The model under review builds one solid part; all positions refer to its coordinate system, in mm. A direction names the side the tool comes from. Round coordinates to 2 decimals unless told otherwise and drop trailing zeros. Write each loop counter-clockwise with the first axis right and the second up, starting at its lowest first coordinate (ties: lowest second). Pieces come first, ordered by that corner, then holes. Notation, with made-up numbers: (58.5, 36) - (92.5, 36) arc R30 cw to (92.5, 60) - close; hole circle Ø11 at (35, 46). An arc over 180 degrees is marked (long way). Return JSON: item names as keys, results as strings.
Autodesk Inventor part; units mm, degrees
ref_plane "YZ Plane" through (0, 0, 0) normal (1, 0, 0) x (0, 1, 0)
ref_plane "XZ Plane" through (0, 0, 0) normal (0, 1, 0) x (-1, 0, 0)
ref_plane "XY Plane" through (0, 0, 0) normal (0, 0, 1) x (1, 0, 0)
sketch "Sketch1" plane through (0, 0, 0) normal (0, 0, 1) x (1, 0, 0)
  line L0 (17.5514, 0) -> (46.0756, 0)
  line L1 (46.0756, 0) -> (46.0756, 12.7)
  line L2 (46.0756, 12.7) -> (0, 12.7)
  line L3 (0, 12.7) -> (0, 0)
  line L4 (17.5514, 12.7) -> (17.5514, 0)
  line L5 (46.0756, 8.9662) -> (42.3672, 8.9662)
  line L6 (42.3672, 7.747) -> (42.3672, 0)
  line L7 (46.0756, 7.747) -> (42.3672, 7.747)
  line L8 (46.0756, 8.9662) -> (42.3672, 7.747)
  line L9 (0, 11.1252) -> (0, 12.7)
  line L10 (17.5514, 0) -> (23.85, 0)
  line L11 (0, -2.5) -> (0, 0)
  line L12 (0, 12.7) -> (38.0365, 12.7)
  line L13 (38.0365, 12.7) -> (38.0365, 14.2748)
  line L14 (38.0365, 14.2748) -> (0, 14.2748)
  line L15 (0, 14.2748) -> (0, 12.7)
  line L16 (17.5514, 12.7) -> (17.5514, 14.2748)
  line L17 (0, 0) -> (17.5514, 0)
  dimension "d1" = 12.7
  dimension "d3" = 3.7338
  dimension "d5" = 4.953
  dimension "d8" = 17.5514
  dimension "d9" = 42.3672
  dimension "d10" = 46.0756
  dimension "d11" = 1.5748
  dimension "d12" = 38.0365
revolve "Revolution1" add sketch "Sketch1" angle 360 about axis through (0, 12.7, 0) along (0, -1, 0) contours L4 L2 L1 L8 L6 L0 | L17 L3 L2 L4 | L16 L14 L13 L2 | L2 L15 L14 L16
sketch "Sketch2" plane through (0, 14.2748, 0) normal (0, 1, 0) x (1, 0, 0)
  circle A0 centre (0, 0) radius 30.1752
  point P0 (0, 30.1752)
  point P1 (0, -30.1752)
  dimension "d14" = 60.3504
hole "Hole1" at (0, 14.2748, -30.1752) at (0, 14.2748, 30.1752) direction (0, -1, 0) diameter 6.35 depth 10.16
properties part number "2016.06.09 Blank Adapter"
(1) Add section A-A (x = 0). Write out the cut boundary in (y, z), plus the area to 3 significant figures.
Filled in:
{"outline": "(0, -42.37) - (7.75, -42.37) - (8.97, -46.08) - (12.7, -46.08) - (12.7, -38.04) - (14.27, -38.04) - (14.27, -33.35) - (4.11, -33.35) - (4.11, -27) - (14.27, -27) - (14.27, 27) - (4.11, 27) - (4.11, 33.35) - (14.27, 33.35) - (14.27, 38.04) - (12.7, 38.04) - (12.7, 46.08) - (8.97, 46.08) - (7.75, 42.37) - (0, 42.37) - close", "area": "1,100 mm2"}
(2) For faces 4 (the cylindrical face through (-9.18, 3.82, -41.36)), 5 (the cylindrical face through (-0.954, 9.124, 33.204)), 6 (the flat face through (-1, 14.275, 1)), list the 3-axis set-ups (+Z, -Z, +X, -X, +Y, -Y) from which the entire face can be reached by the end or side of a thin tool; tool diameter is ignored.
Filled in:
{"face 4": "-Y", "face 5": "+Y", "face 6": "+Z, -Z, +X, -X, +Y"}
(3) Wall thickness on line 1 (Z direction, x = 0, y = 9.25); line 2 (Z direction, x = 0, y = 6.75); line 3 (Y direction, x = 13, z = 39): over which ranges is each line inside the solid? List them lowest first.
Filled in:
{"line 1": "z = -46.08 to -33.35, -27 to 27, 33.35 to 46.08", "line 2": "z = -42.37 to -33.35, -27 to 27, 33.35 to 42.37", "line 3": "y = 0 to 12.7"}
(4) Mouldability with a two-part tool opening along Z and no side actions: class faces 1 (the flat face through (-1, 0, 1)), 2 (the flat face through (0, 4.115, 30)), 3 (the cylindrical face through (-9.99, 10.86, 44.98)) as released by +Z, released by -Z, zero draft, split by the parting line, or undercut.
Filled in:
{"face 1": "zero draft", "face 2": "undercut", "face 3": "split by the parting line"}
(5) Add section B-B (y = 5.5). Write out the cut boundary in (x, z) (3 decimals).
Filled in:
{"outline": "circle Ø84.734 at (0, 0); hole circle Ø6.35 at (0, -30.175); hole circle Ø6.35 at (0, 30.175)"}
(6) Add section C-C (z = 0). Write out the cut boundary in (x, y), plus the area to 3 significant figures.
Filled in:
{"outline": "(-46.08, 8.97) - (-42.37, 7.75) - (-42.37, 0) - (42.37, 0) - (42.37, 7.75) - (46.08, 8.97) - (46.08, 12.7) - (38.04, 12.7) - (38.04, 14.27) - (-38.04, 14.27) - (-38.04, 12.7) - (-46.08, 12.7) - close", "area": "1,230 mm2"}
(7) Clearance check with flat-ended pins moving along their axes: pin 1 Ø8 at (y, z) = (3.5, -18) entering from +X; pin 2 Ø12 at (x, z) = (30, -20.5) entering from -Y; pin 3 Ø3 at (x, z) = (-0.5, 30) entering from +Y; pin 4 Ø1 at (y, z) = (11, -21) entering from -X. State where each tip first meets the part, or that it passes through.
Filled in:
{"pin 1": "stops at x = 39.99", "pin 2": "stops at y = 0", "pin 3": "stops at y = 4.11", "pin 4": "stops at x = -41.26"}
